Can you work these out from the model? Positions are in its coordinate system, mm. Round coordinates to 2 decimals unless told otherwise and drop trailing zeros. Loops run counter-clockwise (first coordinate to the right, second up) from the corner with the lowest first, then second, coordinate; pieces in that order, holes last. Notation, with made-up numbers: (-38, -20) -> (9, -20) arc R20 cw to (9, -6) -> close; hole circle Ø10 at (84, 67.5). An arc over 180 degrees is marked (long way). Write item = value, one per line.
from build123d import *

# Parameters (mm, degrees)
SKETCH1_R          = 55.5
BASE_FLANGE1_DEPTH = 20
FILLET_1_0_R       = 1


# Sheet-metal steps are written as plain solids
with BuildPart() as part:
    # Sketch1 → Base-Flange1 (new body)
    with BuildSketch(Plane(origin=(0, 0, 0), x_dir=(0, 0, -1), z_dir=(1, 0, 0))):
        with BuildLine():
            Line((0, -41), (0, -12.5))
            ThreePointArc((0, -12.5), (3.661165235, -3.661165235), (12.5, 0))
            Line((12.5, 0), (402, 0))
            Line((402, 0), (360.323614104, 222.774084629))
            ThreePointArc((360.323614104, 222.774084629), (305.433470455, 285.831465011), (223.63616123, 268.558327081))
            ThreePointArc((223.63616123, 268.558327081), (88.211160813, 191.873835227), (-67.07058856, 181.480551789))
            ThreePointArc((-67.07058856, 181.480551789), (-155.059207322, 134.23982179), (-133.058215758, 36.825038658))
            Line((-133.058215758, 36.825038658), (-45.972209781, -36.315142143))
            ThreePointArc((-45.972209781, -36.315142143), (-39.95421417, -39.792323471), (-33.109612021, -41))
            Line((-33.109612021, -41), (0, -41))
        make_face()
        with Locations((-80, 100)):
            Circle(SKETCH1_R, mode=Mode.SUBTRACT)
        with Locations((279.230483668, 207.603250897)):
            Circle(SKETCH1_R, mode=Mode.SUBTRACT)
    extrude(amount=-BASE_FLANGE1_DEPTH)

    # Fillet-1.0
    fillet_1_0_edges = [part.edges().sort_by_distance(p)[0] for p in [
        (-10, 0, -402),
        (-10, -41, 0),
    ]]
    fillet(fillet_1_0_edges, radius=FILLET_1_0_R)


solid = part.part
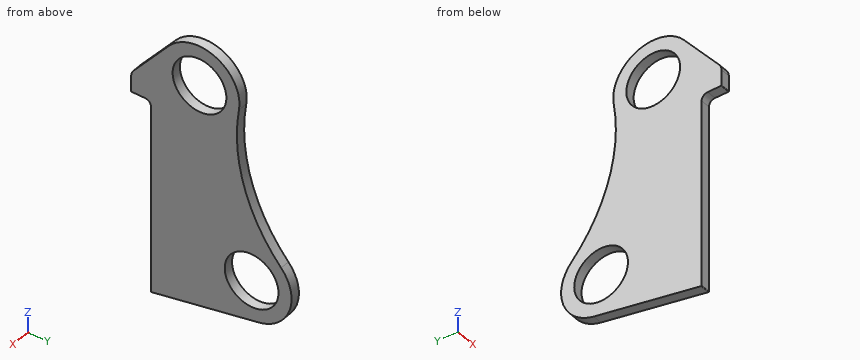
1. Suppose I cut it at A-A, the plane z = 80. List the corners of the cut face in (x, y) for me.
Entries:
outline = (-20, -7.74) -> (0, -7.74) -> (0, 44.5) -> (-20, 44.5) -> close; (-20, 155.5) -> (0, 155.5) -> (0, 182.5) -> (-20, 182.5) -> close
2. Suppose I cut it at D-D, the plane y = 20. List the corners of the cut face in (x, z) for me, and give its area (3 significant figures).
Entries:
outline = (-20, -398.26) -> (0, -398.26) -> (0, 113.03) -> (-20, 113.03) -> close
area = 10,200 mm²
3. Suppose I cut it at C-C, the plane x = -16.75. List the corners of the cut face in (y, z) for me, and give its area (3 significant figures).
Entries:
outline = (-41, 1) arc R1 ccw to (-40, 0) -> (-12.5, 0) arc R12.5 cw to (0, -12.5) -> (0, -400.8) arc R1 ccw to (1.18, -401.78) -> (222.77, -360.32) arc R82.5 ccw to (268.56, -223.64) arc R350 cw to (181.48, 67.07) arc R82.5 ccw to (36.83, 133.06) -> (-36.32, 45.97) arc R20 ccw to (-41, 33.11) -> close; hole circle Ø111 at (100, 80); hole circle Ø111 at (207.6, -279.23)
area = 97,700 mm²
4. I'm going to push flat-ended pins straight in: pin 1 (8 mm diameter, centred on x = -2, z = -223, fed in from +Y); pin 2 (10 mm diameter, centred on x = -9.5, y = -20.5, fed in from -Z); pin 3 (8 mm diameter, centred on x = -2.5, y = 104, fed in from -Z). Where does each tip first touch, or does it pass through?
Entries:
pin_1 = 271.46
pin_2 = 0
pin_3 = -383.29
5. Suppose I cut it at B-B, the plane y = 100. List the corners of the cut face in (x, z) for me.
Entries:
outline = (-20, -383.29) -> (0, -383.29) -> (0, 24.5) -> (-20, 24.5) -> close; (-20, 135.5) -> (0, 135.5) -> (0, 162.5) -> (-20, 162.5) -> close
6. I need wall thicknesses on line 1 (Z direction, x = -10.5, y = 110.5); line 2 (Y direction, x = -6.5, z = -330); line 3 (Y direction, x = -2.5, z = -229). Which ranges of each line are inside material? Lowest first, please. Write a range as [from, to].
Entries:
line_1 = [-381.33, 25.5], [134.5, 161.83]
line_2 = [0, 185.18], [230.02, 272.63]
line_3 = [0, 184], [231.21, 273.05]
